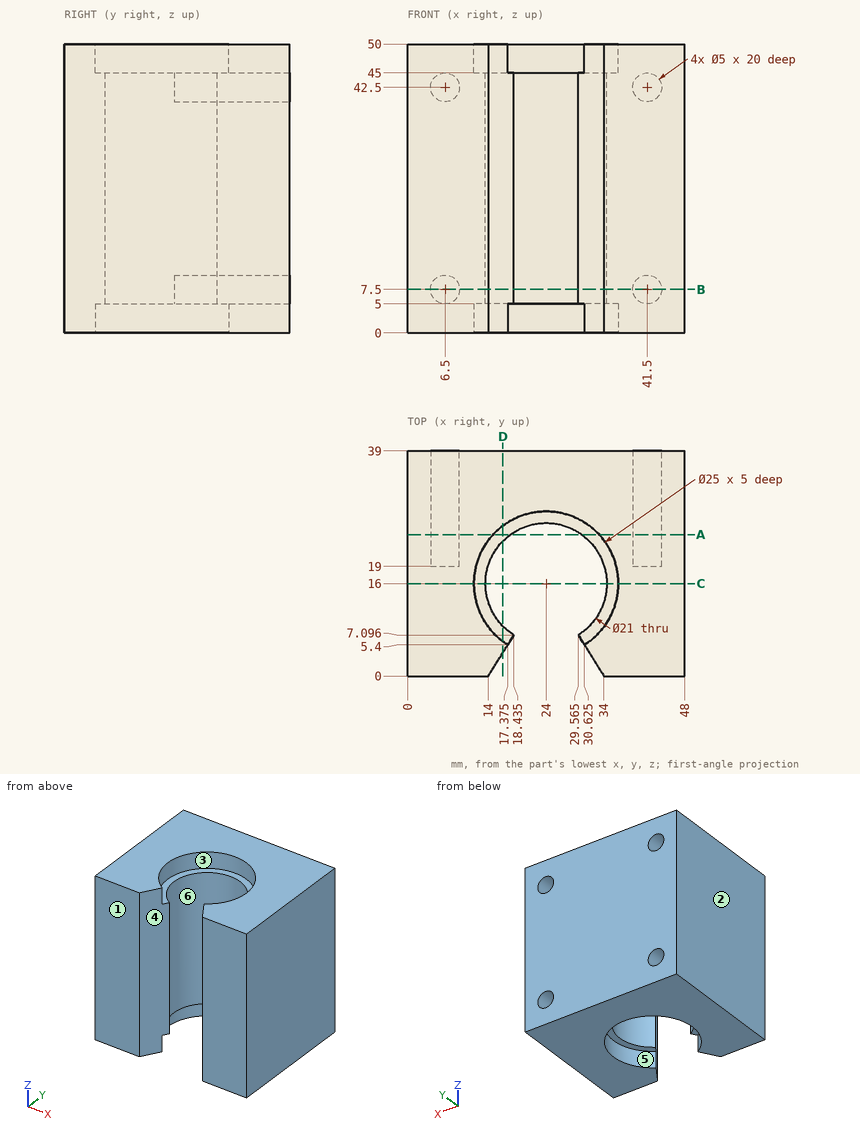
Study the drawing (mm; zero at the part's minimum x, y, z) and answer. A direction names the side the tool comes from. Give positions to 0.01 mm unless a question says otherwise; leave off trailing zeros. Write each loop counter-clockwise with the first axis right and the second up, starting at its lowest first coordinate (ties: lowest second). Pieces come first, ordered by that corner, then holes.
(1) The mould has two halves that part along X. Classify the marked faces 1, 2 and 3: pulls with the +X half, pulls with the -X half, needs draft (parallel to the pull), parting line crosses it, or undercut.
Final values:
face 1: needs draft
face 2: pulls with the -X half
face 3: undercut
(2) Which of the six approach directions +Z, -Z, +X, -X, +Y, -Y give full straight-line access (tool end or side, diameter ignored) to the marked faces 4, 5 and 6?
Final values:
face 4: +Z, -Z, -Y
face 5: -Z
face 6: +Z, -Z
(3) The part is cut by section C-C on y = 16. Write down the section's boundary in (x, z).
Final values:
outline: (0, 0) - (11.5, 0) - (11.5, 5) - (13.5, 5) - (13.5, 45) - (11.5, 45) - (11.5, 50) - (0, 50) - close; (34.5, 5) - (36.5, 5) - (36.5, 0) - (48, 0) - (48, 50) - (36.5, 50) - (36.5, 45) - (34.5, 45) - close
(4) The part is cut by section B-B on z = 7.5. Write down the section's boundary in (x, y) (3 decimals), plus the area to 3 significant figures.
Final values:
outline: (0, 0) - (14, 0) - (18.435, 7.096) arc R10.5 cw (long way) to (29.565, 7.096) - (34, 0) - (48, 0) - (48, 39) - (44, 39) - (44, 19) - (39, 19) - (39, 39) - (9, 39) - (9, 19) - (4, 19) - (4, 39) - (0, 39) - close
area: 1,230 mm2
(5) The part is cut by section D-D on x = 16.5. Write down the section's boundary in (y, z).
Final values:
outline: (4, 0) - (6, 0) - (6, 5) - (8.65, 5) - (8.65, 45) - (6, 45) - (6, 50) - (4, 50) - close; (23.35, 5) - (26, 5) - (26, 0) - (39, 0) - (39, 50) - (26, 50) - (26, 45) - (23.35, 45) - close
(6) Straight lines are drawn through the part: line 1 (Z direction, x = 41.5, y = 31.25); line 2 (X direction, y = 16, z = 48.45); line 3 (Z direction, x = 6, y = 27). For each, find the intervals that lie inside material, in ascending order.
Final values:
line 1: z = 0 to 5, 10 to 40, 45 to 50
line 2: x = 0 to 11.5, 36.5 to 48
line 3: z = 0 to 5.05, 9.95 to 40.05, 44.95 to 50
(7) The part is cut by section A-A on y = 24.5. Write down the section's boundary in (x, z).
Final values:
outline: (0, 0) - (14.83, 0) - (14.83, 5) - (17.84, 5) - (17.84, 45) - (14.83, 45) - (14.83, 50) - (0, 50) - close; (30.16, 5) - (33.17, 5) - (33.17, 0) - (48, 0) - (48, 50) - (33.17, 50) - (33.17, 45) - (30.16, 45) - close; hole circle Ø5 at (6.5, 7.5); hole circle Ø5 at (6.5, 42.5); hole circle Ø5 at (41.5, 7.5); hole circle Ø5 at (41.5, 42.5)
(8) Flat-ended cylindrical pins translate along their axes: pin 1 Ø1.5 at (x, z) = (41.5, 42.5) entering from +Y; pin 2 Ø2 at (x, z) = (17, 12.5) entering from -Y; pin 3 Ø3 at (x, z) = (20, 7) entering from -Y. Find the tip coordinate at first contact, or state that the pin passes through.
Final values:
pin 1: stops at y = 19
pin 2: stops at y = 3.2
pin 3: stops at y = 24.94
